Geometry check sheet. Reference: the model listing, model coordinates, mm. A direction names the side the tool comes from. Coordinates: 2 decimals unless noted, no trailing zeros. Order: outer loops, then holes, each group sorted by start corner. A loop starts at its lowest first (then second) coordinate and runs counter-clockwise, first axis right, second up. Notation, with made-up numbers: (-9, -21.5) - (15, -21.5) arc R20 cw to (15, 5.5) - close; hole circle Ø3 at (-0.75, 30.5). An arc over 180 degrees is marked (long way). Put each result on its own line as item: value.
from build123d import *

# Parameters (mm, degrees)
SKETCH_1_R      = 5.1
SKETCH_1_R_2    = 7.5
SKETCH_1_W      = 5
SKETCH_1_H      = 10
EXTRUDE_1_DEPTH = 5


with BuildPart() as part:
    # 草图1 → 凸台-拉伸1 (new body)
    with BuildSketch(Plane(origin=(0, 0, 0), x_dir=(1, 0, 0), z_dir=(0, 1, 0))):
        with BuildLine():
            Line((5, 0), (75, 0))
            ThreePointArc((75, 0), (78.535533906, 1.464466094), (80, 5))
            Line((80, 5), (80, 21))
            ThreePointArc((80, 21), (81.464466094, 24.535533906), (85, 26))
            Line((85, 26), (95, 26))
            ThreePointArc((95, 26), (98.535533906, 27.464466094), (100, 31))
            Line((100, 31), (100, 38))
            Line((100, 38), (90, 38))
            Line((90, 38), (90, 43))
            Line((90, 43), (70, 43))
            Line((70, 43), (70, 38))
            Line((70, 38), (10, 38))
            Line((10, 38), (10, 43))
            Line((10, 43), (-10, 43))
            Line((-10, 43), (-10, 38))
            Line((-10, 38), (-20, 38))
            Line((-20, 38), (-20, 31))
            ThreePointArc((-20, 31), (-18.535533906, 27.464466094), (-15, 26))
            Line((-15, 26), (-5, 26))
            ThreePointArc((-5, 26), (-1.464466094, 24.535533906), (0, 21))
            Line((0, 21), (0, 5))
            ThreePointArc((0, 5), (1.464466094, 1.464466094), (5, 0))
        make_face()
        with Locations(Location((15, 13, 0), (0, 0, 270))):
            Circle(SKETCH_1_R, mode=Mode.SUBTRACT)
        with Locations(Location((65, 13, 0), (0, 0, 270))):
            Circle(SKETCH_1_R_2, mode=Mode.SUBTRACT)
        with Locations((40, 23)):
            Rectangle(SKETCH_1_W, SKETCH_1_H, mode=Mode.SUBTRACT)
        with BuildLine():
            ThreePointArc((10.242718447, 21.134042717), (8.299573716, 19.625606863), (6.813051963, 17.665646852))
            ThreePointArc((6.813051963, 17.665646852), (7.373585621, 15.619723584), (9.419508889, 16.180257242))
            ThreePointArc((9.419508889, 16.180257242), (10.432770655, 17.516229984), (11.757281553, 18.544429117))
            ThreePointArc((11.757281553, 18.544429117), (12.2948068, 20.59651747), (10.242718447, 21.134042717))
        make_face(mode=Mode.SUBTRACT)
        with BuildLine():
            ThreePointArc((23.134042717, 17.757281553), (21.625606863, 19.700426284), (19.665646852, 21.186948037))
            ThreePointArc((19.665646852, 21.186948037), (17.619723584, 20.626414379), (18.180257242, 18.580491111))
            ThreePointArc((18.180257242, 18.580491111), (19.516229984, 17.567229345), (20.544429117, 16.242718447))
            ThreePointArc((20.544429117, 16.242718447), (22.59651747, 15.7051932), (23.134042717, 17.757281553))
        make_face(mode=Mode.SUBTRACT)
        with BuildLine():
            ThreePointArc((19.757281553, 4.865957283), (21.700426284, 6.374393137), (23.186948037, 8.334353148))
            ThreePointArc((23.186948037, 8.334353148), (22.626414379, 10.380276416), (20.580491111, 9.819742758))
            ThreePointArc((20.580491111, 9.819742758), (19.567229345, 8.483770016), (18.242718447, 7.455570883))
            ThreePointArc((18.242718447, 7.455570883), (17.7051932, 5.40348253), (19.757281553, 4.865957283))
        make_face(mode=Mode.SUBTRACT)
        with BuildLine():
            ThreePointArc((6.865957283, 8.242718447), (8.374393137, 6.299573716), (10.334353148, 4.813051963))
            ThreePointArc((10.334353148, 4.813051963), (12.380276416, 5.373585621), (11.819742758, 7.419508889))
            ThreePointArc((11.819742758, 7.419508889), (10.483770016, 8.432770655), (9.455570883, 9.757281553))
            ThreePointArc((9.455570883, 9.757281553), (7.40348253, 10.2948068), (6.865957283, 8.242718447))
        make_face(mode=Mode.SUBTRACT)
    extrude(amount=EXTRUDE_1_DEPTH)


solid = part.part
Q1. Section check B-B on y = 1.15. State how many separate pieces and enclosed holes the cut face has, then the cut area to 3 significant figures.
Answer block:
separate pieces: 1
enclosed holes: 7
area: 3,320 mm^2
Q2. Thickness scan on L1, parallel to X at y = 3.25, z = -13; L2, parallel to X at y = 3.9, z = -40; L3, parallel to Z at x = 18.5, y = 4.6. Record the ranges inside material, lowest first. Write a range as [from, to].
Answer block:
L1: x = [0, 9.9], [20.1, 57.5], [72.5, 80]
L2: x = [-10, 10], [70, 90]
L3: z = [-38, -21.32], [-18.39, -16.71], [-9.29, -7.61], [-4.75, 0]
Q3. Draft check along Z on faces 1 (the cylindrical face through (19.584, 2.465, -8.501)), 2 (the cylindrical face through (12.31, 2.46, -20.57)), 3 (the cylindrical face through (78, 2, -1)), 4 (the flat face through (100, 2, -34)). Enter one of: pulls with the +Z half, pulls with the -Z half, needs draft (parallel to the pull), parting line crosses it, or undercut.
Answer block:
face 1: undercut
face 2: undercut
face 3: pulls with the +Z half
face 4: needs draft
Q4. Depth check by flat-ended pin: pin 1 Ø1.5 at (y, z) = (1.5, -21) entering from -X; pin 2 Ø1.5 at (y, z) = (1.5, -40) entering from +X; pin 3 Ø2 at (x, y) = (25, 1) entering from -Z. Enter the tip coordinate at first touch or a pass-through.
Answer block:
pin 1: stops at x = -0.06
pin 2: stops at x = 90
pin 3: stops at z = -38
Q5. Access from +Z, -Z, +X, -X, +Y, -Y to the whole of each face (thin tool, end or side, straight path). Record for faces 5 (the flat face through (-10, 2, -26)), 6 (the cylindrical face through (10.416, 2.465, -17.499)), 7 (the flat face through (70, 2, -41)), 8 (the flat face through (90, 2, -26)).
Answer block:
face 5: +Z, -X, +Y, -Y
face 6: +Y, -Y
face 7: -Z, +Y, -Y
face 8: +Z, +X, +Y, -Y
Q6. Section check C-C on x = 15. Record the boundary of the cut face in (y, z), then the cut area to 3 significant figures.
Answer block:
outline: (0, -38) - (5, -38) - (5, -18.1) - (0, -18.1) - close; (0, -7.9) - (5, -7.9) - (5, 0) - (0, 0) - close
area: 139 mm^2
Q7. Section check D-D on x = 35. Record the boundary of the cut face in (y, z).
Answer block:
outline: (0, -38) - (5, -38) - (5, 0) - (0, 0) - close
Q8. Section check A-A on x = 65. Record the boundary of the cut face in (y, z).
Answer block:
outline: (0, -38) - (5, -38) - (5, -20.5) - (0, -20.5) - close; (0, -5.5) - (5, -5.5) - (5, 0) - (0, 0) - close
